```python
from build123d import *

# Parameters (mm, degrees)
F0_R      = 12.7
F1_DEPTH  = 25.4
F1_FACE_R = 12.7
F2_DEPTH  = 19.05
F4_DEPTH  = 1.27
F5_W      = 2.606842
F5_H      = 9.399671
F6_DEPTH  = 1.27


with BuildPart() as f1:
    # F0 (on Front) → F1 (new body)
    with BuildSketch(Plane.XZ):
        Circle(F0_R)
    extrude(amount=F1_DEPTH)

    # F1_face (on face) → F2 (cut)
    with BuildSketch(Plane.XZ.offset(25.4)):
        Circle(F1_FACE_R)
    extrude(amount=-F2_DEPTH, mode=Mode.SUBTRACT)

    # F3 (on face) → F4 (join)
    with BuildSketch(Plane.XZ.offset(6.35)):
        with BuildLine():
            ThreePointArc((-4.587039, 9.399671), (-3.018959, -0.00863), (-4.687303, -9.399671))
            ThreePointArc((-4.687303, -9.399671), (6.518988, -0.0595), (-4.587039, 9.399671))
        make_face()
        with BuildLine():
            ThreePointArc((-3.018959, 8.547434), (4.103795, 0.050131), (-3.018959, -8.447171))
            ThreePointArc((-3.018959, -8.447171), (9.3e-05, 0.050131), (-3.018959, 8.547434))
        make_face(mode=Mode.SUBTRACT)
    extrude(amount=F4_DEPTH)

    # F5 (on face) → F6 (join)
    with BuildSketch(Plane(origin=(0, 0, 0), x_dir=(-1, 0, 0), z_dir=(0, 1, 0))):
        Polygon((-1.228224, 7.895724), (-1.228224, 0), (1.378618, 0), (1.378618, 7.895724), (6.592303, 7.895724), (6.592303, 9.951118), (-6.893092, 9.951118), (-6.893092, 7.895724), align=None)
        with Locations((0.075197, -4.699835)):
            Rectangle(F5_W, F5_H)
    extrude(amount=F6_DEPTH)


solid = f1.part
```
Build history of the part. All positions in model axes, mm. A direction names the side the tool comes from. Give positions to 0.01 mm unless a question says otherwise; leave off trailing zeros. Loops run counter-clockwise (first coordinate to the right, second up) from the corner with the lowest first, then second, coordinate; pieces in that order, holes last.
Item 1: Slice it at D-D, the plane x = 4.75. List the corners of the cut face in (y, z), and give its area (3 significant figures).
Answers follow:
outline: (-7.62, -5.54) - (-6.35, -5.54) - (-6.35, -11.78) - (0, -11.78) - (0, 7.9) - (1.27, 7.9) - (1.27, 9.95) - (0, 9.95) - (0, 11.78) - (-6.35, 11.78) - (-6.35, 5.52) - (-7.62, 5.52) - close
area: 166 mm2
Item 2: Slice it at B-B, the plane z = 0. List the corners of the cut face in (x, y), and give its area (3 significant figures).
Answers follow:
outline: (-12.7, -6.35) - (-3.02, -6.35) - (-3.02, -7.62) - (0, -7.62) - (0, -6.35) - (4.1, -6.35) - (4.1, -7.62) - (6.52, -7.62) - (6.52, -6.35) - (12.7, -6.35) - (12.7, 0) - (1.23, 0) - (1.23, 1.27) - (-1.38, 1.27) - (-1.38, 0) - (-12.7, 0) - close
area: 172 mm2
Item 3: Pull direction Z, two halves, no side cores. Call faces 6 (the face through (-6.592, 1, 9)), 7 (the face through (4, 1, 7.896)), 8 (the face through (-3.02, -6.98, 0.13)): released by +Z, released by -Z, zero draft, split by the parting line, or undercut.
Answers follow:
face 6: zero draft
face 7: released by -Z
face 8: undercut
Item 4: Flat gauge pins, fed straight in: pin 1 (2 mm diameter, centred on x = 1.5, z = 0.5, fed in from -Y); pin 2 (5 mm diameter, centred on x = -9.5, y = -2.5, fed in from +Z); pin 3 (0.6 mm diameter, centred on y = 0.5, z = 0, fed in from +X). Where does each tip first touch, or does it go through?
Answers follow:
pin 1: stops at y = -6.35
pin 2: stops at z = 10.6
pin 3: stops at x = 1.23
Item 5: Drill centre lines: line 1 (Y direction, x = -10, z = -4.5); line 2 (Y direction, x = -2.5, z = 5); line 3 (Z direction, x = -0.25, y = -1.5). Where is each one in solid material? Low to high.
Answers follow:
line 1: y = -6.35 to 0
line 2: y = -7.62 to 0
line 3: z = -12.7 to 12.7
Item 6: Slice it at C-C, the plane y = -4.5. List the corners of the cut face in (x, z).
Answers follow:
outline: circle Ø25.4 at (0, 0)
Item 7: Which spindle directions (+Z, -Z, +X, -X, +Y, -Y) get a long thin tool onto all of the face, cutting with end or side? Do faces 1 (the face through (-4, 1, 7.896)), 2 (the face through (6.893, 1, 9)), 3 (the face through (0, 1, -9.4)), 4 (the face through (-6, -6.35, 0)), 5 (the face through (1.228, 1, -1)). Say none if no direction does.
Answers follow:
face 1: -Z, -X, +Y
face 2: +Z, -Z, +X, +Y
face 3: -Z, +X, -X, +Y
face 4: -Y
face 5: -Z, +X, +Y
Item 8: Slice it at A-A, the plane x = 1.75. List the corners of the cut face in (y, z).
Answers follow:
outline: (-7.62, -8.27) - (-6.35, -8.27) - (-6.35, -12.58) - (0, -12.58) - (0, 7.9) - (1.27, 7.9) - (1.27, 9.95) - (0, 9.95) - (0, 12.58) - (-6.35, 12.58) - (-6.35, 8.25) - (-7.62, 8.25) - (-7.62, 5.97) - (-6.35, 5.97) - (-6.35, -5.87) - (-7.62, -5.87) - close
